from build123d import *

# Parameters (mm, degrees)
F0_R     = 8.5
F1_DEPTH = 25
F2_R     = 2.825
F3_DEPTH = 22
F4_R     = 4.875
F5_DEPTH = 6.5
F6_R     = 6
F7_DEPTH = 3.2
F8_R     = 1.5875
F9_DEPTH = 25


with BuildPart() as f1:
    # F0 (on Top) → F1 (new body)
    with BuildSketch(Plane.XY):
        Circle(F0_R)
    extrude(amount=F1_DEPTH)

    # F2 (on face) → F3 (cut)
    with BuildSketch(Plane.XY.offset(25)):
        Circle(F2_R)
    extrude(amount=-F3_DEPTH, mode=Mode.SUBTRACT)

    # F4 (on face) → F5 (cut)
    with BuildSketch(Plane.XY.offset(25)):
        Circle(F4_R)
    extrude(amount=-F5_DEPTH, mode=Mode.SUBTRACT)

    # F6 (on face) → F7 (cut)
    with BuildSketch(Plane.XY.offset(25)):
        Circle(F6_R)
    extrude(amount=-F7_DEPTH, mode=Mode.SUBTRACT)

    # F8 (on Top) → F9 (join)
    with BuildSketch(Plane.XY):
        with Locations((0, -8.5)):
            Circle(F8_R)
        with Locations((4.996175, -6.876644)):
            Circle(F8_R)
        with Locations((8.08398, -2.626644)):
            Circle(F8_R)
        with Locations((8.08398, 2.626644)):
            Circle(F8_R)
        with Locations((4.996175, 6.876644)):
            Circle(F8_R)
        with Locations((0, 8.5)):
            Circle(F8_R)
        with Locations((-4.996175, 6.876644)):
            Circle(F8_R)
        with Locations((-8.08398, 2.626644)):
            Circle(F8_R)
        with Locations((-8.08398, -2.626644)):
            Circle(F8_R)
        with Locations((-4.996175, -6.876644)):
            Circle(F8_R)
    extrude(amount=F9_DEPTH)


solid = f1.part
Input: part model. Units: mm. Frame: model coordinates. A direction names the side the tool comes from. Give positions to 0.01 mm unless a question says otherwise; leave off trailing zeros. Write each loop counter-clockwise with the first axis right and the second up, starting at its lowest first coordinate (ties: lowest second). Pieces come first, ordered by that corner, then holes.
Q1. Set-up query: faces 3 (the face through (0, -3, 18.5)), 4 (the face through (-5.9, 8.18, 12.32)). Return all of +Z, -Z, +X, -X, +Y, -Y with unobstructed straight access to the full face (end or side cutting, diameter ignored); none if empty.
Q2. Section A-A, the plane y = 0. Output: boundary loops of the cut face in (x, z) (3 decimals).
Q3. Material intervals for probe 1 along Y at (x, z) = (0, 22.5); probe 2 along Y at (x, z) = (0, 14.5) (1 decimal); probe 3 along X at (y, z) = (-0.25, 10.25), sorted ascending.
Q4. Pull-direction query (Y, two-part tool) for faces 1 (the face through (-8.5, 0, 12.3)), 2 (the face through (0, 0, 0)); classes: pulls with the +Y half, pulls with the -Y half, needs draft (parallel to the pull), parting line crosses it, or undercut.
Q5. First-contact query: P1, Ø1.5, axis at y = -7, z = 8.5, coming from the +X side; P2, Ø1.5, axis at x = -1.5, y = -0.5, coming from the +Z side; P3, Ø1, axis at y = -0.5, z = 8, coming from the +X side. Flat tips, straight axial feed; report the tip coordinate or a pass-through.
Q6. Section D-D, the plane x = -3.25. Output: boundary loops of the cut face in (y, z).
Q7. Section C-C, the plane x = 0. Output: boundary loops of the cut face in (y, z) (1 decimal).
Filled in:
1. face 3: +Z
1. face 4: +Z, -Z
2. outline: (-8.5, 0) - (8.5, 0) - (8.5, 25) - (6, 25) - (6, 21.8) - (4.875, 21.8) - (4.875, 18.5) - (2.825, 18.5) - (2.825, 3) - (-2.825, 3) - (-2.825, 18.5) - (-4.875, 18.5) - (-4.875, 21.8) - (-6, 21.8) - (-6, 25) - (-8.5, 25) - close
3. probe 1: y = -10.09 to -6, 6 to 10.09
3. probe 2: y = -10.1 to -2.8, 2.8 to 10.1
3. probe 3: x = -8.5 to -2.81, 2.81 to 8.5
4. face 1: undercut
4. face 2: needs draft
5. P1: stops at x = 6.58
5. P2: stops at z = 3
5. P3: stops at x = 8.5
6. outline: (-7.85, 0) - (7.85, 0) - (7.85, 25) - (5.04, 25) - (5.04, 21.8) - (3.63, 21.8) - (3.63, 18.5) - (-3.63, 18.5) - (-3.63, 21.8) - (-5.04, 21.8) - (-5.04, 25) - (-7.85, 25) - close
7. outline: (-10.1, 0) - (10.1, 0) - (10.1, 25) - (6, 25) - (6, 21.8) - (4.9, 21.8) - (4.9, 18.5) - (2.8, 18.5) - (2.8, 3) - (-2.8, 3) - (-2.8, 18.5) - (-4.9, 18.5) - (-4.9, 21.8) - (-6, 21.8) - (-6, 25) - (-10.1, 25) - close
